Geometry: final body of the model. Coordinates: model frame, mm. Give positions to 0.01 mm unless a question says otherwise; leave off trailing zeros. Order: outer loops, then holes, each group sorted by start corner. A loop starts at its lowest first (then second) coordinate and runs counter-clockwise, first axis right, second up. Notation, with made-up numbers: (88, 75.5) - (107, 75.5) arc R20 ccw to (107, 82.5) - close; hole circle Ø11 at (28.25, 80). An arc over 180 degrees is marked (long way). Write item = value, one per line. Start each with the question number.
Autodesk Inventor part; units mm, degrees
ref_plane "YZ Plane" through (0, 0, 0) normal (1, 0, 0) x (0, 1, 0)
ref_plane "XZ Plane" through (0, 0, 0) normal (0, 1, 0) x (-1, 0, 0)
ref_plane "XY Plane" through (0, 0, 0) normal (0, 0, 1) x (1, 0, 0)
sketch "Sketch1" plane through (0, 0, 0) normal (0, 1, 0) x (-1, 0, 0)
  circle A0 centre (0, 0) radius 6.35
  dimension "d0" = 12.7
extrude "Extrusion1" add sketch "Sketch1" along normal blind 481.6856
sketch "Sketch2" plane through (0, 0, 0) normal (0, -1, 0) x (1, 0, 0)
  point P0 (0, 0)
  point P1 (0, 0)
hole "Hole1" at (0, 0, 0) direction (0, 1, 0) diameter 4.9784 depth 25.4
sketch "Sketch3" plane through (0, 481.6856, 0) normal (0, 1, 0) x (1, 0, 0)
  point P0 (0, 0)
  point P1 (0, 0)
hole "Hole2" at (0, 481.6856, 0) direction (0, -1, 0) diameter 4.9784 depth 25.4
properties part number "Intake BeaterBar" material "Aluminum 7075"
Q1. Section A-A, the plane x = 0. Return the cut outline in (y, z), then the cut area to 3 significant figures.
Q2. Material intervals for line 1 along Z through (x, y) = (0, 471.25); line 2 along X through (y, z) = (76, 0.5); line 3 along Y through (x, z) = (-1.75, -1.25), sorted ascending. Write a range as from..to.
Q3. Section B-B, the plane z = 0. Return the cut outline in (x, y).
Q4. Contact query for flat-ended pins moving along their axis: pin 1 (5 mm diameter, centred on y = 211, z = -5, fed in from -X); pin 2 (4.5 mm diameter, centred on x = 0, z = 0, fed in from +Y); pin 3 (2 mm diameter, centred on y = 194, z = 3, fed in from -X). Output: stop coordinate, or through.
Q5. Section C-C, the plane y = 324. Return the cut outline in (x, z).
The answers:
q1.outline = (0, -6.35) - (481.69, -6.35) - (481.69, -2.49) - (456.29, -2.49) - (456.29, 2.49) - (481.69, 2.49) - (481.69, 6.35) - (0, 6.35) - (0, 2.49) - (25.4, 2.49) - (25.4, -2.49) - (0, -2.49) - close
q1.area = 5,860 mm²
q2.line_1 = -6.35..-2.49, 2.49..6.35
q2.line_2 = -6.33..6.33
q2.line_3 = 25.4..456.29
q3.outline = (-6.35, 0) - (-2.49, 0) - (-2.49, 25.4) - (2.49, 25.4) - (2.49, 0) - (6.35, 0) - (6.35, 481.69) - (2.49, 481.69) - (2.49, 456.29) - (-2.49, 456.29) - (-2.49, 481.69) - (-6.35, 481.69) - close
q4.pin_1 = -5.84
q4.pin_2 = 456.29
q4.pin_3 = -6.03
q5.outline = circle Ø12.7 at (0, 0)
